Drawing for the job (mm, zero at the part's lowest x, y, z). Round coordinates to 2 decimals unless told otherwise and drop trailing zeros. Loops run counter-clockwise (first coordinate to the right, second up) from the corner with the lowest first, then second, coordinate; pieces in that order, holes last. Notation, with made-up numbers: M -37.75,21 L 5.25,21 A32 ccw 5.25,49 Z; hole C 25,80.25 d7. An arc over 180 degrees is marked long. Write each question's results on one line, items separated by ' | '.
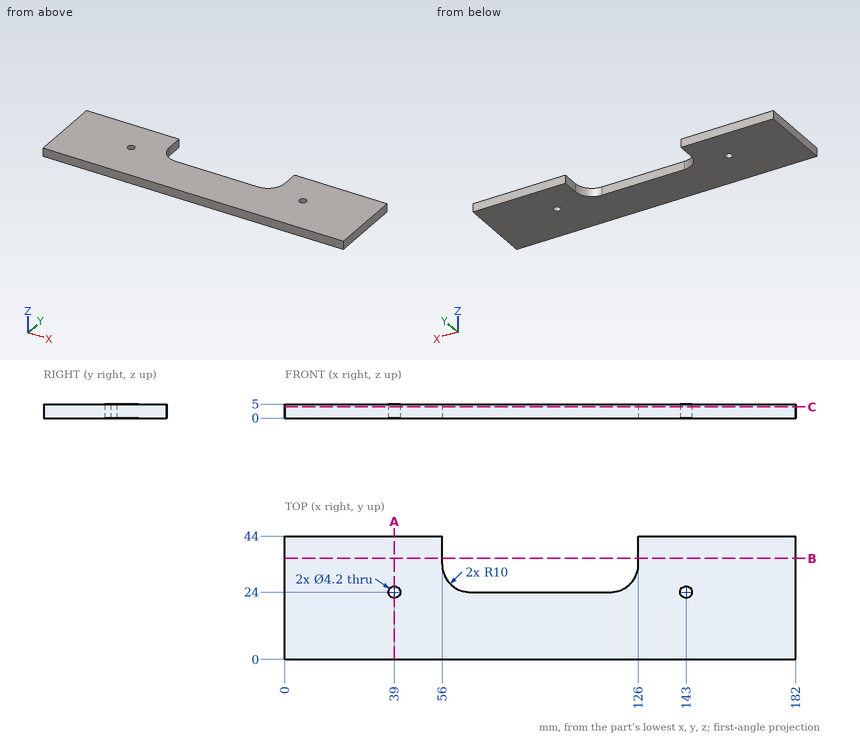
Item 1: Band-saw the part on C-C on z = 3.95. Give the cut face in (x, y).
Filled sheet:
outline: M 0,0 L 182,0 L 182,44 L 126,44 L 126,34 A10 cw 116,24 L 66,24 A10 cw 56,34 L 56,44 L 0,44 Z; hole C 39,24 d4.2; hole C 143,24 d4.2
Item 2: Band-saw the part on A-A on x = 39. Give the cut face in (y, z).
Filled sheet:
outline: M 0,0 L 21.9,0 L 21.9,5 L 0,5 Z; M 26.1,0 L 44,0 L 44,5 L 26.1,5 Z
Item 3: Wall check: L1, parallel to Y at x = 143, z = 2.9; L2, parallel to Y at x = 111, z = 4.2; L3, parallel to X at y = 25, z = 3.4. Give the ranges that are in metal, low to high.
Filled sheet:
L1: 0 to 21.9, 26.1 to 44 | L2: 0 to 24 | L3: 0 to 37.15, 40.85 to 61.64, 120.36 to 141.15, 144.85 to 182
Item 4: Band-saw the part on B-B on y = 36. Give the cut face in (x, z).
Filled sheet:
outline: M 0,0 L 56,0 L 56,5 L 0,5 Z; M 126,0 L 182,0 L 182,5 L 126,5 Z
Item 5: Drop a flat-ended pin along its axis: P1, Ø1.5, axis at x = 97.5, z = 2.5, coming from the +Y side. Give the stop position or say it passes through.
Filled sheet:
P1: y = 24
